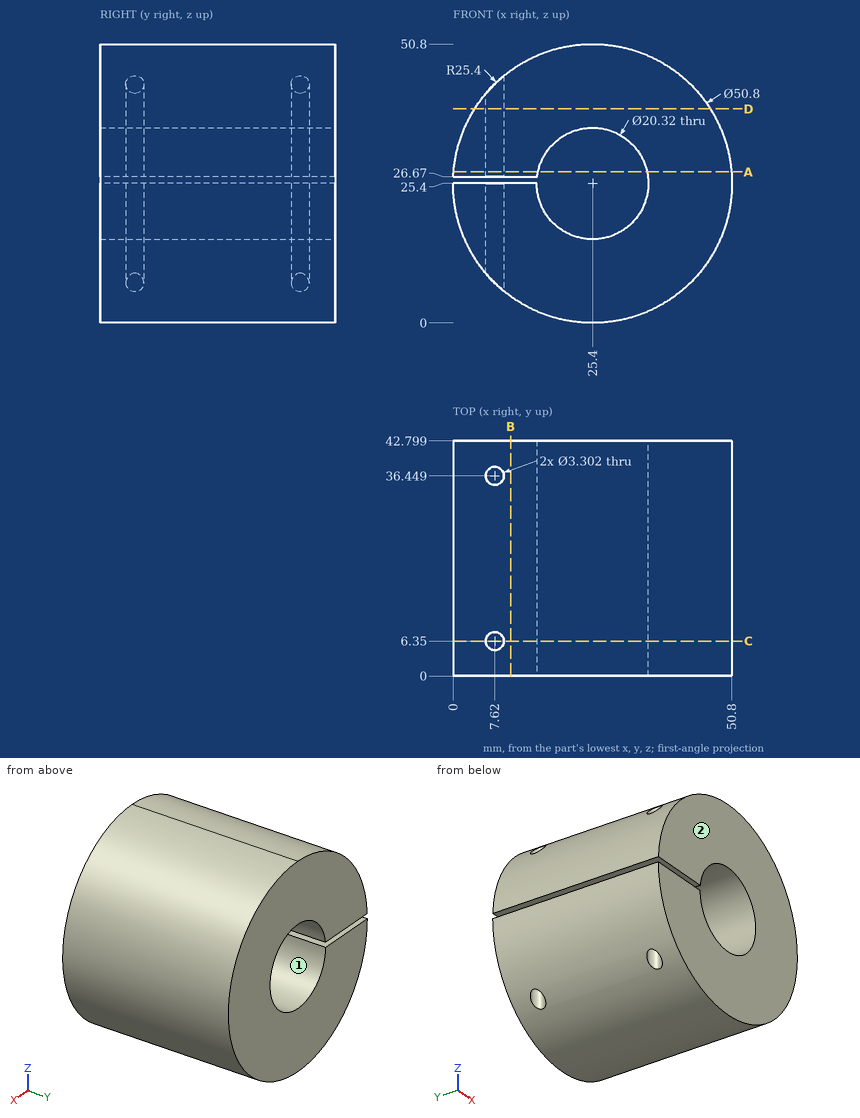
Answer from the drawing. Dimensions are ordinates in mm from the lowest x, y and z of the part. Round coordinates to 2 decimals unless told otherwise and drop trailing zeros. Write each loop counter-clockwise with the first axis right and the second up, starting at its lowest first coordinate (ties: lowest second). Pieces come first, ordered by that corner, then holes. Notation, with made-up numbers: (-12, -5.5) - (25, -5.5) arc R28 ccw to (25, 32.5) - close; hole circle Ø3 at (-34.75, 15). An arc over 180 degrees is marked (long way). Use a Markdown table: item, result.
(1) The part is cut by section C-C (y = 6.35). Write down the section's boundary in (x, z), then the cut area to 3 significant figures.
Reported:
| item | result |
|---|---|
| outline | (0, 25.4) arc R25.4 ccw to (5.97, 9.04) - (5.97, 25.4) - close; (0.03, 26.67) - (5.97, 26.67) - (5.97, 41.76) arc R25.4 ccw to start; (9.27, 5.78) arc R25.4 ccw (long way) to (9.27, 45.02) - (9.27, 26.67) - (15.32, 26.67) arc R10.16 cw (long way) to (15.24, 25.4) - (9.27, 25.4) - close |
| area | 1,570 mm2 |
(2) Straight lines are drawn through the part: line 1 along Y through (x, z) = (7.62, 39); line 2 along X through (y, z) = (6, 20); line 3 along X through (y, z) = (12.5, 16). For each, find the intervals that lie inside material, in ascending order. Write a range as [from, to].
Reported:
| item | result |
|---|---|
| line 1 | [0, 4.7], [8, 34.8], [38.1, 42.8] |
| line 2 | [0.58, 6.01], [9.23, 16.79], [34.01, 50.22] |
| line 3 | [1.8, 21.54], [29.26, 49] |
(3) The mould has two halves that part along X. Classify the marked faces 1 and 2: released by +X, released by -X, zero draft, split by the parting line, or undercut.
Reported:
| item | result |
|---|---|
| face 1 | undercut |
| face 2 | zero draft |
(4) The part is cut by section B-B (x = 10.5). Write down the section's boundary in (y, z).
Reported:
| item | result |
|---|---|
| outline | (0, 4.83) - (42.8, 4.83) - (42.8, 25.4) - (0, 25.4) - close; (0, 26.67) - (42.8, 26.67) - (42.8, 45.97) - (0, 45.97) - close |
(5) The part is cut by section A-A (z = 27.5). Write down the section's boundary in (x, y), then the cut area to 3 significant figures.
Reported:
| item | result |
|---|---|
| outline | (0.09, 0) - (15.46, 0) - (15.46, 42.8) - (0.09, 42.8) - close; (35.34, 0) - (50.71, 0) - (50.71, 42.8) - (35.34, 42.8) - close; hole circle Ø3.3 at (7.62, 6.35); hole circle Ø3.3 at (7.62, 36.45) |
| area | 1,300 mm2 |
(6) The part is cut by section D-D (z = 39). Write down the section's boundary in (x, y), then the cut area to 3 significant figures.
Reported:
| item | result |
|---|---|
| outline | (3.95, 0) - (46.85, 0) - (46.85, 42.8) - (3.95, 42.8) - close; hole circle Ø3.3 at (7.62, 6.35); hole circle Ø3.3 at (7.62, 36.45) |
| area | 1,820 mm2 |
(7) Each of these flat-tipped pins is pushed along its axis until it touches: pin 1 Ø4.5 at (x, y) = (11, 14) entering from +Z; pin 2 Ø1.5 at (x, y) = (6.5, 35) entering from -Z; pin 3 Ø10 at (x, z) = (33.5, 30.5) entering from -Y; pin 4 Ø4 at (y, z) = (8, 29) entering from +X. Where does it stop, or does it pass through?
Reported:
| item | result |
|---|---|
| pin 1 | z = 47.71 |
| pin 2 | z = 7.65 |
| pin 3 | y = 0 |
| pin 4 | x = 50.75 |
